```python
from build123d import *

# Parameters (mm, degrees)
F0_W      = 1270
F0_H      = 1270
F1_DEPTH  = 304.8
F2_W      = 355.16951
F2_H      = 1270
F3_DEPTH  = 609.6
F4_R      = 87.321685
F5_DEPTH  = 660.4
F6_W      = 86.208582
F6_H      = 414.878845
F6_W_2    = 96.984655
F6_H_2    = 441.819012
F7_DEPTH  = 127
F8_W      = 135.951609
F8_H      = 651.744328
F8_W_2    = 117.517472
F8_H_2    = 622.415811
F9_DEPTH  = 127
F11_DEPTH = 381
F12_W     = 89.866299
F12_H     = 336.422592
F13_DEPTH = 25.4
F14_W     = 295.283154
F14_H     = 1175.713479
F15_DEPTH = 647.7
F17_DEPTH = 508


with BuildPart() as f1:
    # F0 (on Front) → F1 (new body)
    with BuildSketch(Plane.XZ):
        with Locations((-0.384308, 25.70168)):
            Rectangle(F0_W, F0_H)
    extrude(amount=F1_DEPTH)

    # F2 (on Top) → F3 (join)
    with BuildSketch(Plane.XY):
        with Locations((8.173354, -683.127984)):
            Rectangle(F2_W, F2_H)
    extrude(amount=-F3_DEPTH)

    # F4 (on Top) → F5 (join)
    with BuildSketch(Plane.XY):
        with Locations((0, -530.925989)):
            Circle(F4_R)
    extrude(amount=-F5_DEPTH)

    # F6 (on Front) → F7 (join)
    with BuildSketch(Plane.XZ):
        with Locations((419.371635, -520.395398)):
            Rectangle(F6_W, F6_H)
        with Locations((-386.139914, -533.865482)):
            Rectangle(F6_W_2, F6_H_2)
    extrude(amount=F7_DEPTH)

    # F8 (on Top) → F9 (join)
    with BuildSketch(Plane.XY):
        with Locations((401.709839, -396.605987)):
            Rectangle(F8_W, F8_H)
        with Locations((-370.218724, -411.270245)):
            Rectangle(F8_W_2, F8_H_2)
    extrude(amount=-F9_DEPTH)

    # F10 (on Front) → F11 (cut)
    with BuildSketch(Plane.XZ):
        Polygon((-627.267778, 274.273783), (0, 663.457155), (-627.267778, 663.457155), align=None)
        Polygon((0, 663.457155), (634.537637, 274.273783), (643.659174, 663.457155), align=None)
    extrude(amount=F11_DEPTH, mode=Mode.SUBTRACT)

    # F12 (on Front) → F13 (join)
    with BuildSketch(Plane.XZ):
        with Locations((3.072093, -36.667466)):
            Rectangle(F12_W, F12_H)
    extrude(amount=-F13_DEPTH)

    # F14 (on Right) → F15 (join)
    with BuildSketch(Plane.YZ):
        with Locations((-191.560142, 71.131975)):
            Rectangle(F14_W, F14_H)
    extrude(amount=F15_DEPTH)

    # F16 (on Front) → F17 (cut)
    with BuildSketch(Plane.XZ):
        Polygon((628.30925, 654.611826), (0, 666.133165), (628.30925, 274.408251), align=None)
    extrude(amount=F17_DEPTH, mode=Mode.SUBTRACT)


solid = f1.part
```
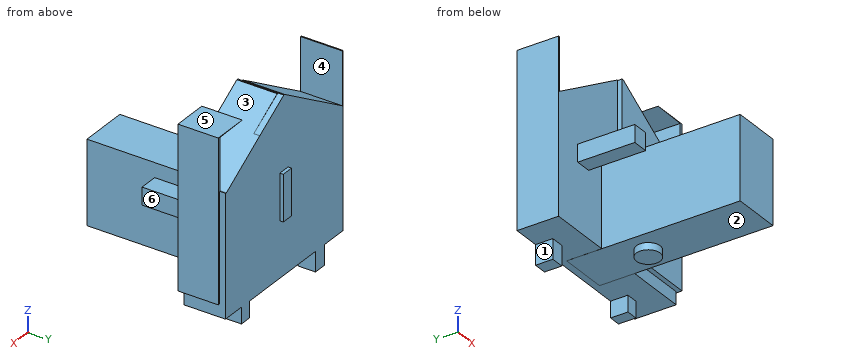
Geometry: final body of the model. Coordinates: model frame, mm. Face numbers are marked on the shaded views. A direction names the side the tool comes from. Round coordinates to 2 decimals unless told otherwise and drop trailing zeros. Order: outer loops, then holes, each group sorted by start corner. A loop starts at its lowest first (then second) coordinate and runs counter-clockwise, first axis right, second up. Notation, with made-up numbers: M 55.5,11.5 L 75.5,11.5 A21 cw 75.5,23.5 Z; hole C 43,-1.5 d2. An arc over 180 degrees is marked long. Use one line per item in the form item = value. Start each with the question number.
Q1. Material intervals for line 1 (X direction, y = -406, z = -42); line 2 (Z direction, x = -98.5, y = -384); line 3 (Z direction, x = -374, y = -617.5), sorted ascending. Write a range as [from, to].
Q2. Cut plane D-D (z = 26). Return loops of the section in (x, y), and give its area (3 significant figures).
Q3. Mould query, pull axis Z, two halves, no side actions, for the marked faces 1, 2 and 3. Classes: +Z half, -Z half, draft (parallel to the pull), parting line (faces both ways), or undercut.
Q4. Access query for the marked faces 4, 5 and 6. Directions: +Z, -Z, +X, -X, +Y, -Y. A direction counts if a zero-diameter tool reaches every point of the face in a straight line with its end or side. Return the directions, or none.
Q5. Cut plane C-C (z = 424). Return loops of the section in (x, y).
Q6. Cut plane B-B (y = -217). Return loops of the section in (x, z).
Q7. Cut plane A-A (z = 200). Return loops of the section in (x, y).
Q8. Pin query (flat end, axial travel): pin 1 Ø4 at (y, z) = (-1080.5, -393) entering from -X; pin 2 Ø6 at (x, y) = (-258.5, -147.5) entering from +Z; pin 3 Ø3 at (x, z) = (-188, 74.5) entering from -Y. Return the tip coordinate at first contact, or that it passes through.
Geometry results:
q1.line_1 = [-428.98, -311.46], [-169.41, 185.76], [333.73, 469.69]
q1.line_2 = [-609.6, 0]
q1.line_3 = [-127, 0]
q2.outline = M -635.38,-304.8 L 0,-304.8 L 0,-339.2 L 647.7,-339.2 L 647.7,-43.92 L 634.62,-43.92 L 634.62,0 L 48.01,0 L 48.01,25.4 L -41.86,25.4 L -41.86,0 L -635.38,0 Z
q2.area = 415,000 mm^2
q3.face_1 = draft
q3.face_2 = -Z half
q3.face_3 = undercut
q4.face_4 = +Z, +Y, -Y
q4.face_5 = +Z, +X, +Y, -Y
q4.face_6 = +Z, -Z, +X, -Y
q5.outline = M -635.38,-304.8 L -627.27,-304.8 L -627.27,0 L -635.38,0 Z; M -385.95,-304.8 L 0,-304.8 L 0,-339.2 L 388.37,-339.2 L 388.37,0 L -385.95,0 Z; M 628.31,-339.2 L 647.7,-339.2 L 647.7,-43.92 L 628.31,-43.92 Z
q6.outline = M -635.38,-609.3 L -169.41,-609.3 L -169.41,-609.6 L 185.76,-609.6 L 185.76,-609.3 L 634.62,-609.3 L 634.62,-516.72 L 647.7,-516.72 L 647.7,658.99 L 389.62,658.99 L 628.31,654.61 L 628.31,274.41 L 11.46,658.99 L 7.29,658.99 L 4.49,660.7 L -4.44,660.7 L -627.27,274.27 L -627.27,660.7 L -635.38,660.7 Z
q7.outline = M -635.38,-304.8 L 0,-304.8 L 0,-339.2 L 647.7,-339.2 L 647.7,-43.92 L 634.62,-43.92 L 634.62,0 L -635.38,0 Z
q8.pin_1 = -169.41
q8.pin_2 = 504.93
q8.pin_3 = -304.8
